Autodesk Fusion 360 part; units mm, degrees
sketch "草图1" plane through (0, 0, 0) normal (1, 0, 0) x (0, 1, 0)
  line L0 (0, 90) -> (0, -60) construction
  line L1 (0, 30) -> (22, 30)
  line L2 (22, 30) -> (22, -30)
  line L3 (22, -30) -> (0, -30)
  line L4 (22, 6) -> (142, 6)
  line L5 (142, 6) -> (142, 17.5)
  line L6 (142, 17.5) -> (161, 17.5)
  line L7 (161, -17.5) -> (142, -17.5)
  line L8 (142, -17.5) -> (142, -6)
  line L9 (142, -6) -> (22, -6)
  line L10 (0, 30) -> (0, -30)
  line L11 (-55, 0) -> (190, 0) construction
  line L12 (161, -17.5) -> (161, -13.4)
  line L13 (161, -13.4) -> (149, -9.2681)
  line L14 (149, -9.2681) -> (149, -2.9268)
  line L15 (149, -2.9268) -> (157.5, 0)
  line L16 (157.5, 0) -> (149, 2.9268)
  line L17 (149, 2.9268) -> (149, 9.2681)
  line L18 (149, 9.2681) -> (161, 13.4)
  line L19 (161, 13.4) -> (161, 17.5)
  line L20 (149, -6.0974) -> (142, -6.0974) construction
  line L21 (149, 6.0974) -> (148, 6.0974)
  line L22 (148, 6.0974) -> (142, 6.0974) construction
  point P0 (149, 6.0974)
  point P1 (149, -6.0974)
  dimension "d1" = 22
  dimension "d2" = 60
  dimension "d3" = 12
  dimension "d5" = 161
  dimension "d6" = 157.5
  dimension "d7" = 149
  dimension "d8" = 13.4
  dimension "d9" = 38
  dimension "d10" = 142
  dimension "d11" = 35
revolve "旋转1" add sketch "草图1" angle 360 about axis through (0, 0, 90) along (0, 0, -1)
sketch "草图2" plane through (0, 0, 6) normal (0, 0, 1) x (-1, 0, 0)
  circle A0 centre (0, 0) radius 22
  circle A1 centre (0, 0) radius 142
  circle A2 centre (0, -90) radius 30
  circle A3 centre (77.9423, -45) radius 30
  circle A4 centre (77.9423, 45) radius 30
  circle A5 centre (0, 90) radius 30
  circle A6 centre (-77.9423, 45) radius 30
  circle A7 centre (-77.9423, -45) radius 30
  dimension "d13" = 90
  dimension "d14" = 60
  dimension "d16" = 360
extrude "拉伸1" cut sketch "草图2" against normal blind 90 contours A2 | A3 | A4 | A5 | A6 | A7
sketch "草图3" plane through (0, 0, 30) normal (0, 0, 1) x (-1, 0, 0)
  circle A0 centre (0, 0) radius 22
  line L0 (3, -9.5394) -> (3, -13.5)
  line L1 (3, -13.5) -> (-3, -13.5)
  line L2 (-3, -13.5) -> (-3, -9.5394)
  line L3 (0, -30) -> (0, 30) construction
  arc A1 (3, -9.5394) -> (-3, -9.5394) centre (0, 0) ccw
  dimension "d19" = 6
  dimension "d20" = 20
  dimension "d21" = 23.5
extrude "拉伸2" cut sketch "草图3" against normal blind 110 contours L0 L1 L2 A1
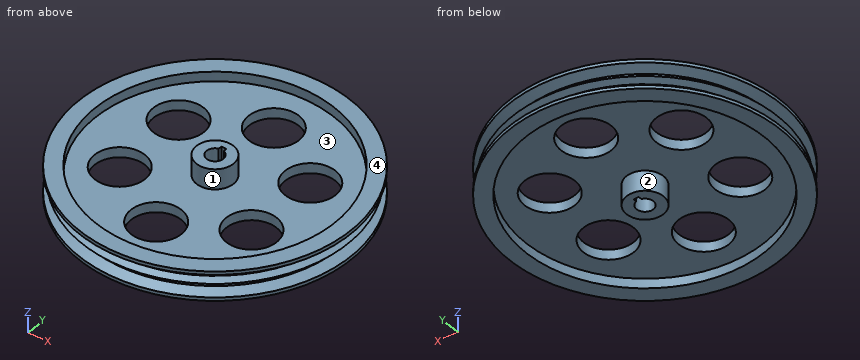
The listing builds one solid part. Answer for the finished solid, in the listing's coordinates (mm). Face numbers are marked on the shaded views. A direction names the side the tool comes from. Give positions to 0.01 mm unless a question says otherwise; leave off trailing zeros. Order: outer loops, then holes, each group sorted by start corner. A loop starts at its lowest first (then second) coordinate and runs counter-clockwise, first axis right, second up. Notation, with made-up numbers: (55, 68.25) - (103, 68.25) arc R34 cw to (103, 107.25) - close; hole circle Ø10 at (-31, 77). An arc over 180 degrees is marked (long way). Answer in a Markdown table with one row per item. Add a question column.
Q1. Given P1, Ø18, axis at x = 0, y = 0, coming from the -Z side; P2, Ø1.2, axis at y = 12, z = -13.5, coming from the -X side; P3, Ø2, axis at x = -74, y = 99, coming from the -Z side; P4, Ø1.5, axis at x = 113.5, z = 8.5, coming from the -Y side, each flat-ended and moving along its own axis, determine where each tip first touches the part or whether it passes through.
Q2. Which of the six approach directions +Z, -Z, +X, -X, +Y, -Y give full straight-line access (tool end or side, diameter ignored) to the marked faces 1 and 2?
Q3. For a pull along X with two mould halves and no side action, classify the marked faces 3 and 4 as released by +X, released by -X, zero draft, split by the parting line, or undercut.
Q4. Find the intervals of material crossed by line 1 along X through (y, z) = (0, -14); line 2 along Z through (x, y) = (101.5, 114); line 3 along Z through (x, y) = (-133.5, -77), in increasing order. Write a range as [from, to].
Q5. The part is cut by section B-B (y = -52). Give the number of separate pieces and of enclosed holes in the cut face, then the cut area to 3 significant figures.
Q6. The part is cut by section A-A (z = -23). Determine the outline of the cut face in (x, y), then the cut area to 3 significant figures.
Determined:
| question | item | result |
|---|---|---|
| 1 | P1 | passes through |
| 1 | P2 | stops at x = -160.6 |
| 1 | P3 | stops at z = -6 |
| 1 | P4 | stops at y = -97.41 |
| 2 | face 1 | +Z |
| 2 | face 2 | -Z |
| 3 | face 3 | undercut |
| 3 | face 4 | zero draft |
| 4 | line 1 | x = [-161, -142], [-22, -10], [10, 22], [142, 161] |
| 4 | line 2 | z = [-17.5, -10.52], [-1.67, 1.67], [10.52, 17.5] |
| 4 | line 3 | z = [-17.5, -11.03], [-1.17, 1.17], [11.03, 17.5] |
| 5 | separate pieces | 3 |
| 5 | enclosed holes | 0 |
| 5 | area | 2,660 mm² |
| 6 | outline | circle Ø44 at (0, 0); hole (-3, 9.54) arc R10 ccw (long way) to (3, 9.54) - (3, 13.5) - (-3, 13.5) - close |
| 6 | area | 1,180 mm² |
